For this review, take the finished solid that the model builds, in its own axes (mm). A direction names the side the tool comes from. Give positions to 0.01 mm unless a question says otherwise; leave off trailing zeros. Order: outer loops, then holes, each group sorted by start corner. A loop starts at its lowest first (then second) coordinate and runs counter-clockwise, first axis right, second up.
Item 1: For P1, Ø6, axis at x = 7.5, y = 3.5, coming from the +Z side; P2, Ø4, axis at x = 8, y = 10.5, coming from the +Z side; P3, Ø2.5, axis at x = 14.5, y = 7.5, coming from the -Z side, all flat-tipped, find the tip position at first contact; note any pin that passes through.
Item 2: The part is to be moulded in two halves that separate along Y. For faces 3 (the cylindrical face through (13.026, 6.148, 6.69)), 4 (the flat face through (14, 0, 4)), 5 (the cylindrical face through (0.9, 7.6, 0.85)), 6 (the flat face through (14, 15, 4)), say which applies: released by +Y, released by -Y, zero draft, split by the parting line, or undercut.
Item 3: Machinability: for faces 1 (the cylindrical face through (18.853, 7.605, 4.283)), 2 (the flat face through (14, 13, 0)), which of the approach directions +Z, -Z, +X, -X, +Y, -Y give a long, thin tool a straight path to every point of the face, cutting with its end or side? Answer none if there is none.
Item 4: Consider section C-C (y = 7.5). Give the boundary of the cut face in (x, z).
Item 5: For probe 1 along X at (y, z) = (11.75, 10.5); probe 2 along X at (y, z) = (7.5, 9); probe 3 along X at (y, z) = (9.25, 8.5), list the stretches that pass through material, from the lowest coordinate up.
Item 6: Consider section A-A (z = 9.5). Give the boundary of the cut face in (x, y).
Item 7: Consider section B-B (x = 14.5). Give the boundary of the cut face in (y, z).
Item 8: Consider section D-D (z = 3.75). Give the boundary of the cut face in (x, y).
```python
from build123d import *

# Parameters (mm, degrees)
SKETCH_W      = 29
SKETCH_H      = 15
PAD_DEPTH     = 3
SKETCH001_W   = 2
SKETCH001_H   = 15
SKETCH001_W_2 = 6
PAD001_DEPTH  = 8
FILLET_R      = 4.5
SKETCH002_R   = 2
POCKET_DEPTH  = 11.001
CHAMFER_SIZE  = 2.5
FILLET001_R   = 2.99


with BuildPart() as part:
    # Sketch → Pad (new body)
    with BuildSketch(Plane.XY):
        with Locations((14.5, 7.5)):
            Rectangle(SKETCH_W, SKETCH_H)
    extrude(amount=PAD_DEPTH)

    # Sketch001 (on Face6 of Pad) → Pad001 (join)
    with BuildSketch(Plane.XY.offset(3)):
        with Locations((1, 7.5)):
            Rectangle(SKETCH001_W, SKETCH001_H)
        with Locations((14.5, 7.5)):
            Rectangle(SKETCH001_W_2, SKETCH001_H)
        with Locations((28, 7.5)):
            Rectangle(SKETCH001_W, SKETCH001_H)
    extrude(amount=PAD001_DEPTH)

    # Fillet
    fillet_edges = [part.edges().sort_by_distance(p)[0] for p in [
        (2, 7.5, 3),
        (11.5, 7.5, 3),
        (17.5, 7.5, 3),
        (27, 7.5, 3),
    ]]
    fillet(fillet_edges, radius=FILLET_R)

    # Sketch002 (on Face6 of Fillet) → Pocket (cut, through all)
    with BuildSketch(Plane(origin=(0, 0, 0), x_dir=(1, 0, 0), z_dir=(0, 0, -1))):
        with Locations((14.5, -7.5)):
            Circle(SKETCH002_R)
    extrude(amount=-POCKET_DEPTH, mode=Mode.SUBTRACT)

    # Chamfer
    chamfer_edges = [part.edges().sort_by_distance(p)[0] for p in [
        (12.5, 7.5, 0),
    ]]
    chamfer(chamfer_edges, length=CHAMFER_SIZE)

    # Fillet001
    fillet001_edges = [part.edges().sort_by_distance(p)[0] for p in [
        (0, 7.5, 0),
        (29, 7.5, 0),
    ]]
    fillet(fillet001_edges, radius=FILLET001_R)


solid = part.part
```
Resolved:
1. P1: stops at z = 4.67
1. P2: stops at z = 4.15
1. P3: passes through
2. face 3: undercut
2. face 4: released by -Y
2. face 5: zero draft
2. face 6: released by +Y
3. face 1: +Z, +Y, -Y
3. face 2: -Z, +X, -X, +Y, -Y
4. outline: (0, 2.99) arc R2.99 ccw to (2.99, 0) - (10, 0) - (12.5, 2.5) - (12.5, 11) - (11.5, 11) - (11.5, 7.5) arc R4.5 cw to (7, 3) - (6.5, 3) arc R4.5 cw to (2, 7.5) - (2, 11) - (0, 11) - close; (16.5, 2.5) - (19, 0) - (26.01, 0) arc R2.99 ccw to (29, 2.99) - (29, 11) - (27, 11) - (27, 7.5) arc R4.5 cw to (22.5, 3) - (22, 3) arc R4.5 cw to (17.5, 7.5) - (17.5, 11) - (16.5, 11) - close
5. probe 1: x = 0 to 2, 11.5 to 17.5, 27 to 29
5. probe 2: x = 0 to 2, 11.5 to 12.5, 16.5 to 17.5, 27 to 29
5. probe 3: x = 0 to 2, 11.5 to 13.53, 15.47 to 17.5, 27 to 29
6. outline: (0, 0) - (2, 0) - (2, 15) - (0, 15) - close; (11.5, 0) - (17.5, 0) - (17.5, 15) - (11.5, 15) - close; (27, 0) - (29, 0) - (29, 15) - (27, 15) - close; hole circle Ø4 at (14.5, 7.5)
7. outline: (0, 0) - (3, 0) - (5.5, 2.5) - (5.5, 11) - (0, 11) - close; (9.5, 2.5) - (12, 0) - (15, 0) - (15, 11) - (9.5, 11) - close
8. outline: (0, 0) - (4.01, 0) - (4.01, 15) - (0, 15) - close; (9.49, 0) - (19.51, 0) - (19.51, 15) - (9.49, 15) - close; (24.99, 0) - (29, 0) - (29, 15) - (24.99, 15) - close; hole circle Ø4 at (14.5, 7.5)
